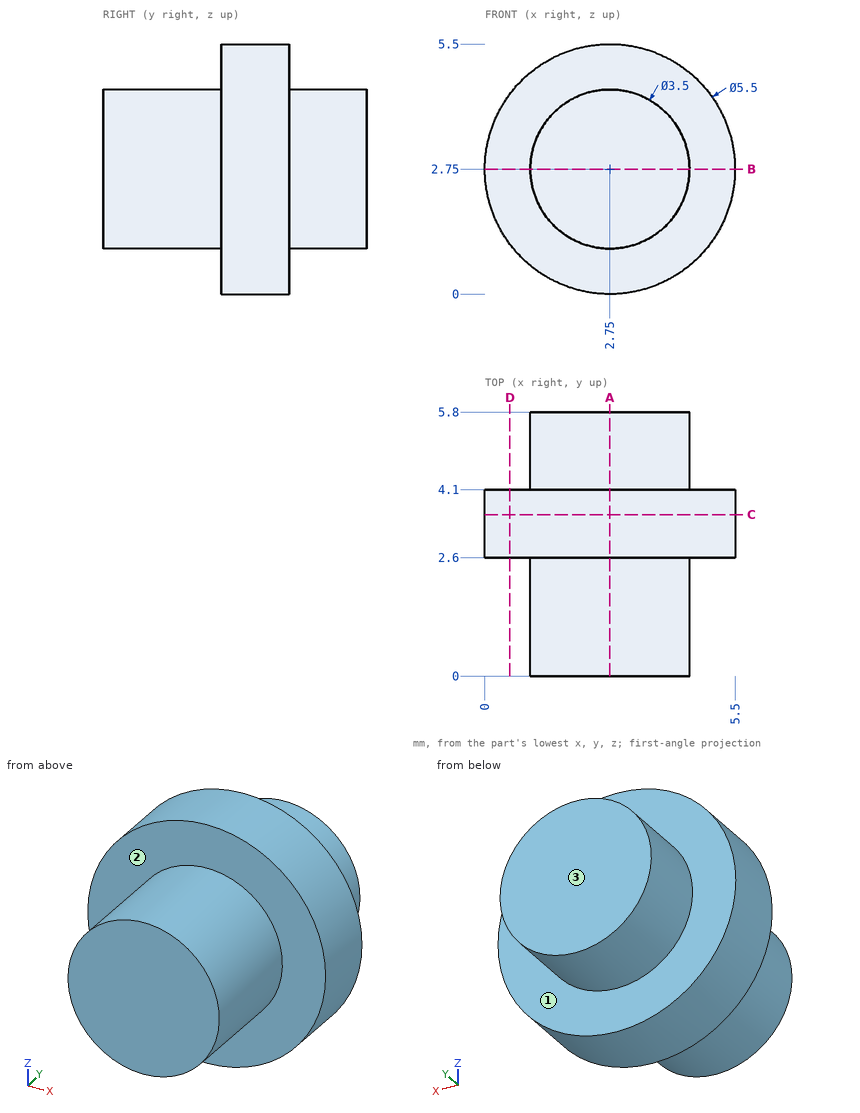
Geometry check sheet. Reference: drawing and pictorial views, mm from the part's lowest x, y, z. A direction names the side the tool comes from. Round coordinates to 2 decimals unless told otherwise and drop trailing zeros. Write each loop counter-clockwise with the first axis right and the second up, starting at its lowest first coordinate (ties: lowest second). Pieces come first, ordered by that corner, then holes. Notation, with made-up numbers: (58, -15) -> (76, -15) arc R9 cw to (76, 2) -> close; hole circle Ø9 at (69, 12.25). An arc over 180 degrees is marked (long way). One line per question, with ' | ' between items. Start each with the question number.
1. Set-up check for the marked faces 1, 2 and 3: record each of +Z, -Z, +X, -X, +Y, -Y from which the full face is reachable in a straight line by a thin tool's end or side.
2. Sectioned sample at C-C, the plane y = 3.55. Record the cut outline in (x, z).
3. Scan lines: line 1 along Y through (x, z) = (4.2, 1.2); line 2 along X through (y, z) = (1.3, 2); line 3 along X through (y, z) = (5.6, 4.2). Record each from-to range of solid material in increasing order. Write a range as from..to.
4. Sectioned sample at D-D, the plane x = 0.55. Record the cut outline in (y, z), then the cut area to 3 significant figures.
5. Sectioned sample at A-A, the plane x = 2.75. Record the cut outline in (y, z), then the cut area to 3 significant figures.
6. Sectioned sample at B-B, the plane z = 2.75. Record the cut outline in (x, y).
7. Depth check by flat-ended pin: pin 1 (1 mm diameter, centred on y = 1.5, z = 2, fed in from +X). Enter the tip coordinate at first touch or a pass-through.
Taken from the geometry:
1) face 1: +Y | face 2: -Y | face 3: +Z, -Z, +X, -X, +Y
2) outline: circle Ø5.5 at (2.75, 2.75)
3) line 1: y = 2.6..4.1 | line 2: x = 1.17..4.33 | line 3: x = 1.77..3.73
4) outline: (2.6, 1.1) -> (4.1, 1.1) -> (4.1, 4.4) -> (2.6, 4.4) -> close | area: 4.95 mm^2
5) outline: (0, 1) -> (2.6, 1) -> (2.6, 0) -> (4.1, 0) -> (4.1, 1) -> (5.8, 1) -> (5.8, 4.5) -> (4.1, 4.5) -> (4.1, 5.5) -> (2.6, 5.5) -> (2.6, 4.5) -> (0, 4.5) -> close | area: 23.3 mm^2
6) outline: (0, 2.6) -> (1, 2.6) -> (1, 0) -> (4.5, 0) -> (4.5, 2.6) -> (5.5, 2.6) -> (5.5, 4.1) -> (4.5, 4.1) -> (4.5, 5.8) -> (1, 5.8) -> (1, 4.1) -> (0, 4.1) -> close
7) pin 1: stops at x = 4.48
